Could you check a few things on this model? Use its own coordinates, in mm. Face numbers are marked on the shaded views. A direction names the side the tool comes from. Coordinates: 2 decimals unless noted, no trailing zeros. Loops run counter-clockwise (first coordinate to the right, second up) from the corner with the lowest first, then second, coordinate; pieces in that order, holes last. Notation, with made-up numbers: (24, 53.5) -> (59, 53.5) arc R17 cw to (59, 63.5) -> close; hole circle Ø8 at (87.5, -3). An arc over 180 degrees is marked (long way). One line per question, with ' | ' between items.
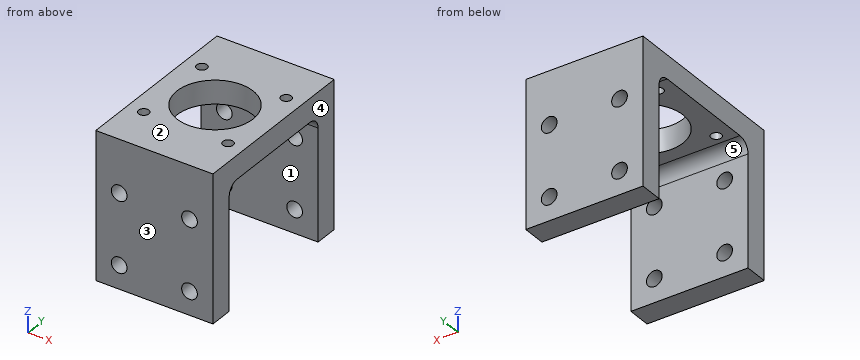
from build123d import *

# Parameters (mm, degrees)
SKETCH1_W               = 25.4
SKETCH1_H               = 38.1
SKETCH1_R               = 8.255
SKETCH1_R_2             = 1.1303
BOSS_EXTRUDE1_DEPTH     = 15.875
CUT_EXTRUDE1_REACH      = 37.498
SKETCH3_W               = 26.67
SKETCH3_H               = 27.94
FILLET1_R               = 2.54
SKETCH5_R               = 1.7
FRAME_MOUNT_HOLES_DEPTH = 44.184668865


with BuildPart() as part:
    # Sketch1 → Boss-Extrude1 (new, symmetric)
    with BuildSketch(Plane.XY):
        Rectangle(SKETCH1_W, SKETCH1_H)
        Circle(SKETCH1_R, mode=Mode.SUBTRACT)
        with Locations((-9.1313, 9.1313)):
            Circle(SKETCH1_R_2, mode=Mode.SUBTRACT)
        with Locations((9.1313, 9.1313)):
            Circle(SKETCH1_R_2, mode=Mode.SUBTRACT)
        with Locations((-9.1313, -9.1313)):
            Circle(SKETCH1_R_2, mode=Mode.SUBTRACT)
        with Locations((9.1313, -9.1313)):
            Circle(SKETCH1_R_2, mode=Mode.SUBTRACT)
    extrude(amount=BOSS_EXTRUDE1_DEPTH, both=True)

    # Sketch3 → Cut-Extrude1 (cut, up to next)
    with BuildSketch(Plane(origin=(12.7, 0, 0), x_dir=(0, 0, -1), z_dir=(1, 0, 0)), mode=Mode.PRIVATE) as cut_extrude1_sk1:
        with Locations((2.54, 0)):
            Rectangle(SKETCH3_W, SKETCH3_H)
    cut_extrude1_tool1 = extrude(cut_extrude1_sk1.sketch, amount=-CUT_EXTRUDE1_REACH, mode=Mode.PRIVATE) & part.part
    add(cut_extrude1_tool1.solids().sort_by_distance((12.7, 0, -2.54))[0], mode=Mode.SUBTRACT)

    # Fillet1
    fillet1_edges = [part.edges().sort_by_distance(p)[0] for p in [
        (0, -13.97, 10.795),
        (0, 13.97, 10.795),
    ]]
    fillet(fillet1_edges, radius=FILLET1_R)

    # Sketch5 → Frame Mount Holes (cut, through all)
    with BuildSketch(Plane(origin=(0, 19.05, 0), x_dir=(1, 0, 0), z_dir=(0, 1, 0))):
        with Locations(Location((-7.62, 10.795, 0), (0, 0, 270))):
            Circle(SKETCH5_R)
        with Locations(Location((-7.62, -4.445, 0), (0, 0, 270))):
            Circle(SKETCH5_R)
        with Locations(Location((7.62, -4.445, 0), (0, 0, 270))):
            Circle(SKETCH5_R)
        with Locations(Location((7.62, 10.795, 0), (0, 0, 270))):
            Circle(SKETCH5_R)
    extrude(amount=-FRAME_MOUNT_HOLES_DEPTH, mode=Mode.SUBTRACT)


solid = part.part
1) If we section it at B-B on y = 0: Please give me the cut outline in (x, z) (3 decimals).
Data:
outline: (-12.7, 10.795) -> (-8.255, 10.795) -> (-8.255, 15.875) -> (-12.7, 15.875) -> close; (8.255, 10.795) -> (12.7, 10.795) -> (12.7, 15.875) -> (8.255, 15.875) -> close
2) I'm going to push flat-ended pins straight in: pin 1 Ø2 at (x, z) = (-7.62, 4.445) entering from -Y; pin 2 Ø2.5 at (x, y) = (-9.13, 9.13) entering from -Z (3 decimals). Where does each tip first touch, or does it pass through?
Data:
pin 1: through | pin 2: z = 10.795
3) If we section it at A-A on x = 0: Please give me the cut outline in (y, z) (3 decimals).
Data:
outline: (-19.05, -15.875) -> (-13.97, -15.875) -> (-13.97, 8.255) arc R2.54 cw to (-11.43, 10.795) -> (-8.255, 10.795) -> (-8.255, 15.875) -> (-19.05, 15.875) -> close; (8.255, 10.795) -> (11.43, 10.795) arc R2.54 cw to (13.97, 8.255) -> (13.97, -15.875) -> (19.05, -15.875) -> (19.05, 15.875) -> (8.255, 15.875) -> close
4) On a 3-axis mill with a long thin cutter (end or side, diameter ignored), from which of +Z, -Z, +X, -X, +Y, -Y can I reach the whole of each face in a straight line? I mean the marked faces 1 and 2. Say none if no direction works.
Data:
face 1: -Z, +X, -X | face 2: +Z, +X, -X, +Y, -Y
5) We'd pull the mould along Y, two halves only. Please class the marked faces 3, 4 and 5: pulls with the +Y half, pulls with the -Y half, needs draft (parallel to the pull), parting line crosses it, or undercut.
Data:
face 3: pulls with the -Y half | face 4: needs draft | face 5: undercut
6) If we section it at C-C on z = 11.5: Please give me the cut outline in (x, y) (3 decimals).
Data:
outline: (-12.7, -19.05) -> (12.7, -19.05) -> (12.7, 19.05) -> (-12.7, 19.05) -> close; hole circle Ø2.261 at (-9.131, -9.131); hole circle Ø2.261 at (-9.131, 9.131); hole circle Ø16.51 at (0, 0); hole circle Ø2.261 at (9.131, -9.131); hole circle Ø2.261 at (9.131, 9.131)
7) I need wall thicknesses on line 1 along Y through (x, z) = (-6.5, -8.5); line 2 along X through (y, z) = (-14.5, -11.5); line 3 along Z through (x, y) = (8.25, -7) (3 decimals). Which ranges of each line are inside material? Lowest first, please. Write a range as from..to.
Data:
line 1: -19.05..-13.97, 13.97..19.05 | line 2: -12.7..-9.17, -6.07..6.07, 9.17..12.7 | line 3: 10.795..15.875
8) If we section it at D-D on y = -16: Please give me the cut outline in (x, z) (3 decimals).
Data:
outline: (-12.7, -15.875) -> (12.7, -15.875) -> (12.7, 15.875) -> (-12.7, 15.875) -> close; hole circle Ø3.4 at (-7.62, -10.795); hole circle Ø3.4 at (-7.62, 4.445); hole circle Ø3.4 at (7.62, -10.795); hole circle Ø3.4 at (7.62, 4.445)
